Geometry check sheet. Reference: the model listing, model coordinates, mm. Face numbers are marked on the shaded views. A direction names the side the tool comes from. Give positions to 0.01 mm unless a question says otherwise; leave off trailing zeros. Loops run counter-clockwise (first coordinate to the right, second up) from the corner with the lowest first, then second, coordinate; pieces in that order, holes last. Notation, with made-up numbers: (10.25, 28) -> (59.25, 28) arc R18 ccw to (59.25, 58) -> close; hole circle Ø9 at (86, 63.25). An arc over 180 degrees is marked (long way). One line per item, written item: value. Start each with the question number.
(1) Sectioned sample at B-B, the plane y = 4.5. Record the cut outline in (x, z), then the cut area to 3 significant figures.
(2) Gauge pin test, flat ends, axial feed: pin 1 Ø2 at (y, z) = (4.5, 4.5) entering from +X; pin 2 Ø1.6 at (x, y) = (0.5, 6) entering from +Z; pin 3 Ø2 at (y, z) = (6.5, 6) entering from -X. Record the tip position at first contact, or that the pin passes through.
(3) Draft check along Z on the marked faces 6, 7, 8 and 9. Enter one of: pulls with the +Z half, pulls with the -Z half, needs draft (parallel to the pull), parting line crosses it, or undercut.
(4) Scan lines: line 1 along X through (y, z) = (4.75, 7.5); line 2 along Z through (x, y) = (-0.5, 1.75); line 3 along X through (y, z) = (1, 12.5). Record each from-to range of solid material in increasing order. Write a range as from..to.
(5) Sectioned sample at C-C, the plane x = -2. Record the cut outline in (y, z).
(6) Sectioned sample at D-D, the plane z = 14.75. Record the cut outline in (x, y).
(7) Sectioned sample at A-A, the plane y = 2. Record the cut outline in (x, z).
(8) Tool access check on the marked faces 1, 2, 3, 4 and 5. Record the directions out of +Z, -Z, +X, -X, +Y, -Y that give a thin tool (end or side, any length) a straight path to the whole face; none if there is none.
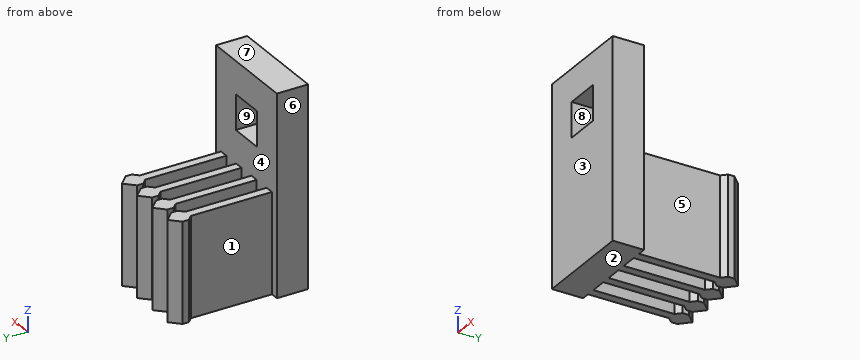
from build123d import *

# Parameters (mm, degrees)
RESSALTO_EXTRUS_O1_DEPTH = 8
ESBO_O4_W                = 8
ESBO_O4_H                = 2.5
RESSALTO_EXTRUS_O3_DEPTH = 8
ESBO_O5_W                = 2.8
ESBO_O5_H                = 2.8
CORTE_EXTRUS_O1_DEPTH    = 20.632180215


with BuildPart() as part:
    # Esboço1 → Ressalto-extrusão1 (new body)
    with BuildSketch(Plane.XY):
        Polygon((0.65, 2.5), (-0.65, 2.5), (-0.65, 9), (-0.25, 9.4), (-0.25, 9.9), (-0.75, 10.4), (-1, 10.65), (-1.25, 10.4), (-1.75, 9.9), (-1.75, 9.4), (-1.35, 9), (-1.35, 2.5), (-2.65, 2.5), (-2.65, 9), (-2.25, 9.4), (-2.25, 9.9), (-2.75, 10.4), (-3, 10.65), (-3.25, 10.4), (-3.75, 9.9), (-3.75, 9.4), (-3.35, 9), (-3.35, 2.5), (-4, 2.5), (-4, 0), (4, 0), (4, 2.5), (3.35, 2.5), (3.35, 9), (3.75, 9.4), (3.75, 9.9), (3.25, 10.4), (3, 10.65), (2.75, 10.4), (2.25, 9.9), (2.25, 9.4), (2.65, 9), (2.65, 2.5), (1.35, 2.5), (1.35, 9), (1.75, 9.4), (1.75, 9.9), (1.25, 10.4), (1, 10.65), (0.75, 10.4), (0.25, 9.9), (0.25, 9.4), (0.65, 9), align=None)
    extrude(amount=RESSALTO_EXTRUS_O1_DEPTH)

    # Esboço4 → Ressalto-extrusão3 (add)
    with BuildSketch(Plane.XY.offset(8)):
        with Locations((0, 1.25)):
            Rectangle(ESBO_O4_W, ESBO_O4_H)
    extrude(amount=RESSALTO_EXTRUS_O3_DEPTH)

    # Esboço5 → Corte-extrusão1 (cut, through all)
    with BuildSketch(Plane.XZ):
        with Locations((0, 12)):
            Rectangle(ESBO_O5_W, ESBO_O5_H)
    extrude(amount=-CORTE_EXTRUS_O1_DEPTH, mode=Mode.SUBTRACT)


solid = part.part
Calculated:
1. outline: (-3.35, 0) -> (-2.65, 0) -> (-2.65, 8) -> (-3.35, 8) -> close; (-1.35, 0) -> (-0.65, 0) -> (-0.65, 8) -> (-1.35, 8) -> close; (0.65, 0) -> (1.35, 0) -> (1.35, 8) -> (0.65, 8) -> close; (2.65, 0) -> (3.35, 0) -> (3.35, 8) -> (2.65, 8) -> close
1. area: 22.4 mm2
2. pin 1: stops at x = 3.35
2. pin 2: stops at z = 8
2. pin 3: stops at x = -3.35
3. face 6: needs draft
3. face 7: pulls with the +Z half
3. face 8: undercut
3. face 9: undercut
4. line 1: x = -3.35..-2.65, -1.35..-0.65, 0.65..1.35, 2.65..3.35
4. line 2: z = 0..10.6, 13.4..16
4. line 3: x = -4..-1.4, 1.4..4
5. outline: (0, 0) -> (2.5, 0) -> (2.5, 16) -> (0, 16) -> close
6. outline: (-4, 0) -> (4, 0) -> (4, 2.5) -> (-4, 2.5) -> close
7. outline: (-4, 0) -> (4, 0) -> (4, 16) -> (-4, 16) -> close; hole (-1.4, 10.6) -> (1.4, 10.6) -> (1.4, 13.4) -> (-1.4, 13.4) -> close
8. face 1: +Z, -Z, -X
8. face 2: -Z, +X, -X, +Y, -Y
8. face 3: +Z, -Z, +X, -X, -Y
8. face 4: +Z
8. face 5: +Z, -Z, +X
